Read the model definition and answer for the solid it produces. Units are mm, in the model's axes. Give positions to 0.01 mm unless a question says otherwise; leave off trailing zeros. Order: outer loops, then holes, each group sorted by start corner. A loop starts at its lowest first (then second) coordinate and runs counter-clockwise, first axis right, second up. Notation, with made-up numbers: M -11.5,-9.5 L -7.5,-9.5 A10 cw -7.5,8.5 Z; hole C 33.25,2.5 d11. An arc over 180 degrees is marked long. One line per item, written item: value.
from build123d import *


with BuildPart() as part:
    # Sketch1 → Revolve3 (revolve)
    with BuildSketch(Plane.XY, mode=Mode.PRIVATE) as revolve3_sk:
        with BuildLine():
            Line((31.75, 495.3), (44.45, 495.3))
            Line((44.45, 495.3), (44.45, 469.9))
            ThreePointArc((44.45, 469.9), (40.730256121, 460.919743879), (31.75, 457.2))
            Line((31.75, 457.2), (-31.75, 457.2))
            ThreePointArc((-31.75, 457.2), (-40.730256121, 460.919743879), (-44.45, 469.9))
            Line((-44.45, 469.9), (-44.45, 495.3))
            Line((-44.45, 495.3), (-31.75, 495.3))
            ThreePointArc((-31.75, 495.3), (0, 478.260567419), (31.75, 495.3))
        make_face()
    revolve(revolve3_sk.sketch.rotate(Axis((0, 0, 0), (-1, 0, 0)), 90), axis=Axis((0, 0, 0), (-1, 0, 0)))


solid = part.part
1) Find section A-A, the plane y = 0. Write down the section's boundary in (x, z).
Reported:
outline: M -44.45,-495.3 L -31.75,-495.3 A38.1 cw 31.75,-495.3 L 44.45,-495.3 L 44.45,-469.9 A12.7 ccw 31.75,-457.2 L -31.75,-457.2 A12.7 ccw -44.45,-469.9 Z; M -44.45,469.9 A12.7 ccw -31.75,457.2 L 31.75,457.2 A12.7 ccw 44.45,469.9 L 44.45,495.3 L 31.75,495.3 A38.1 cw -31.75,495.3 L -44.45,495.3 Z
2) Find section C-C, the plane x = 6. Write down the section's boundary in (y, z).
Reported:
outline: C 0,0 d957.47; hole C 0,0 d914.4
3) Each of these flat-tipped pins is pushed along its axis until it touches: pin 1 Ø12 at (x, z) = (11.5, 247) entering from -Y; pin 2 Ø5 at (x, z) = (-7, 326) entering from -Y; pin 3 Ø4 at (x, y) = (-21.5, -124) entering from -Z. Where does it stop, or does it pass through?
Reported:
pin 1: stops at y = -416.02
pin 2: stops at y = -353.23
pin 3: stops at z = -470.38
4) Determine the mould class of faces 1 (the face through (38.189, 483.522, 107.371)), 2 (the face through (-0.444, -20.102, 456.758)), 3 (the face through (44.45, -369.2, -291.2)) for opening direction Y: +Y half, -Y half, draft (parallel to the pull), parting line (faces both ways), or undercut.
Reported:
face 1: parting line
face 2: undercut
face 3: draft
5) Consider probe 1 along Y at (x, z) = (17.5, 177); probe 2 along Z at (x, y) = (-30.5, 14.5); probe 3 along Y at (x, z) = (9, 0). Determine where each line is inside the solid, lowest interval first.
Reported:
probe 1: y = -448.88 to -421.55, 421.55 to 448.88
probe 2: z = -493.31 to -456.97, 456.97 to 493.31
probe 3: y = -479.34 to -457.2, 457.2 to 479.34
